```python
from build123d import *

# Parameters (mm, degrees)
BOX001_W       = 10
BOX001_H       = 10
BOX001_DEPTH   = 8
CYLINDER_R     = 2.5
CYLINDER_DEPTH = 5
BOX_W          = 16
BOX_H          = 16
BOX_DEPTH      = 10


with BuildPart() as cube001:
    # Box001 → Box001 (new body)
    with BuildSketch(Plane(origin=(-5, -5, 0), x_dir=(1, 0, 0), z_dir=(0, 0, 1))):
        with Locations((5, 5)):
            Rectangle(BOX001_W, BOX001_H)
    extrude(amount=BOX001_DEPTH)


with BuildPart() as cylinder:
    # Cylinder → Cylinder (new body)
    with BuildSketch(Plane.XY.offset(10)):
        Circle(CYLINDER_R)
    extrude(amount=CYLINDER_DEPTH)


with BuildPart() as sphere:
    # Sphere → Sphere (revolve)
    with BuildSketch(Plane(origin=(0, 0, 15), x_dir=(1, 0, 0), z_dir=(0, -1, 0))):
        with BuildLine():
            ThreePointArc((0, -5), (5, 0), (0, 5))
            Line((0, 5), (0, -5))
        make_face()
    revolve(axis=Axis((0, 0, 15), (0, 0, 1)))


with BuildPart() as cut:
    # Box → Box (new body)
    with BuildSketch(Plane(origin=(-8, -8, 0), x_dir=(1, 0, 0), z_dir=(0, 0, 1))):
        with Locations((8, 8)):
            Rectangle(BOX_W, BOX_H)
    extrude(amount=BOX_DEPTH)

    # Fusion: union Cylinder, Sphere
    add(cylinder.part)
    add(sphere.part)

    # Cut: cut Cube001
    add(cube001.part, mode=Mode.SUBTRACT)


solid = cut.part
```
The model under review builds one solid part; all positions refer to its coordinate system, in mm. A direction names the side the tool comes from. Give positions to 0.01 mm unless a question says otherwise; leave off trailing zeros. Write each loop counter-clockwise with the first axis right and the second up, starting at its lowest first coordinate (ties: lowest second). Pieces come first, ordered by that corner, then holes.
(1) For P1, Ø1, axis at y = 2, z = 16, coming from the -X side; P2, Ø5, axis at x = -5.5, y = -0.5, coming from the -Z side; P3, Ø1, axis at x = -0.5, z = 17, coming from the -Y side, all flat-tipped, find the tip position at first contact; note any pin that passes through.
(2) Consider section C-C, the plane z = 15. Give the boundary of the cut face in (x, y), and give its area (3 significant figures).
(3) Consider section B-B, the plane x = 0. Give the boundary of the cut face in (y, z), and give its area (3 significant figures).
(4) Consider section A-A, the plane y = 3. Give the boundary of the cut face in (x, z).
(5) Tool access review of faces 5 (the flat face through (-8, 0, 5)), 6 (the flat face through (-2, 2, 10)), 7 (the flat face through (0, -5, 4)): name each direction out of +Z, -Z, +X, -X, +Y, -Y from which nothing blocks a thin tool from reaching the whole face with its end or side.
(6) To check wall thickness, follow L1, parallel to X at y = -2.5, z = 4.75; L2, parallel to Z at x = 5.25, y = 2.75. State the ranges of each line that lie inside material, in increasing order.
(7) The part is to be moulded in two halves that separate along X. For faces 1 (the flat face through (8, 0, 5)), 2 (the flat face through (0, 8, 5)), 3 (the flat face through (-5, 0, 4)), 4 (the flat face through (5, 0, 4)), say which applies: released by +X, released by -X, zero draft, split by the parting line, or undercut.
(8) Consider section D-D, the plane y = -2. Give the boundary of the cut face in (x, z).
Returned:
1. P1: stops at x = -4.69
1. P2: stops at z = 0
1. P3: stops at y = -4.75
2. outline: circle Ø10 at (0, 0)
2. area: 78.5 mm2
3. outline: (-8, 0) - (-5, 0) - (-5, 8) - (5, 8) - (5, 0) - (8, 0) - (8, 10) - (2.5, 10) - (2.5, 10.67) arc R5 ccw (long way) to (-2.5, 10.67) - (-2.5, 10) - (-8, 10) - close
3. area: 160 mm2
4. outline: (-8, 0) - (-5, 0) - (-5, 8) - (5, 8) - (5, 0) - (8, 0) - (8, 10) - (-8, 10) - close; circle Ø8 at (0, 15)
5. face 5: +Z, -Z, -X, +Y, -Y
5. face 6: none
5. face 7: -Z
6. L1: x = -8 to -5, 5 to 8
6. L2: z = 0 to 10
7. face 1: released by +X
7. face 2: zero draft
7. face 3: undercut
7. face 4: undercut
8. outline: (-8, 0) - (-5, 0) - (-5, 8) - (5, 8) - (5, 0) - (8, 0) - (8, 10) - (1.5, 10) - (1.5, 10.67) arc R4.58 ccw (long way) to (-1.5, 10.67) - (-1.5, 10) - (-8, 10) - close
